Can you work these out from the model? Positions are in its coordinate system, mm. Round coordinates to 2 decimals unless told otherwise and drop trailing zeros. Loops run counter-clockwise (first coordinate to the right, second up) from the corner with the lowest first, then second, coordinate; pieces in that order, holes last.
from build123d import *

# Parameters (mm, degrees)
BOSS_EXTRUDE1_DEPTH = 30
FILLET1_R           = 5
SKETCH2_R           = 14
CUT_EXTRUDE1_DEPTH  = 56.541044473


with BuildPart() as part:
    # Sketch1 → Boss-Extrude1 (new body)
    with BuildSketch(Plane.XY):
        Polygon((0, 40), (34.641016151, -20), (-34.641016151, -20), align=None)
    extrude(amount=BOSS_EXTRUDE1_DEPTH)

    # Fillet1
    fillet1_edges = [part.edges().sort_by_distance(p)[0] for p in [
        (0, 40, 15),
        (34.641016151, -20, 15),
        (-34.641016151, -20, 15),
    ]]
    fillet(fillet1_edges, radius=FILLET1_R)

    # Sketch2 → Cut-Extrude1 (cut, through all)
    with BuildSketch(Plane.XY.offset(30)):
        Circle(SKETCH2_R)
    extrude(amount=-CUT_EXTRUDE1_DEPTH, mode=Mode.SUBTRACT)


solid = part.part
(1) If we section it at D-D, the plane x = 19: List the corners of the cut face in (y, z) for me, then the cut area to 3 significant figures.
Worked answers:
outline: (-20, 0) - (7.09, 0) - (7.09, 30) - (-20, 30) - close
area: 813 mm2
(2) If I drill on line 1 (Y direction, x = 0, z = 9.25); line 2 (Y direction, x = -1, z = 23.5); line 3 (X direction, y = -13, z = 6.5), over which ranges is the centre line in solid material (lowest first)?
Worked answers:
line 1: y = -20 to -14, 14 to 35
line 2: y = -20 to -13.96, 13.96 to 34.9
line 3: x = -30.56 to -5.2, 5.2 to 30.56
(3) If we section it at A-A, the plane x = 0: List the corners of the cut face in (y, z) for me.
Worked answers:
outline: (-20, 0) - (-14, 0) - (-14, 30) - (-20, 30) - close; (14, 0) - (35, 0) - (35, 30) - (14, 30) - close
(4) If we section it at B-B, the plane z = 2: List the corners of the cut face in (x, y) for me, then the cut area to 3 significant figures.
Worked answers:
outline: (-30.31, -12.5) arc R5 ccw to (-25.98, -20) - (25.98, -20) arc R5 ccw to (30.31, -12.5) - (4.33, 32.5) arc R5 ccw to (-4.33, 32.5) - close; hole circle Ø28 at (0, 0)
area: 1,410 mm2
(5) Will these pins go through, and if not, where does the flat tip stop? P1, Ø5, axis at x = 18.5, z = 5.5, coming from the +Y side; P2, Ø1, axis at y = -4, z = 8, coming from the -X side; P3, Ø12, axis at y = 14, z = 5.5, coming from the +X side.
Worked answers:
P1: stops at y = 12.29
P2: stops at x = -25.69
P3: stops at x = 18.48
(6) If we mould it in two halves opening along X, with no side actions, what happens to faces 1 (the flat face through (17.14, 10.31, 14.79)), 2 (the cylindrical face through (-30.274, -17.563, 15.21)), 3 (the cylindrical face through (12.932, -5.362, 15.21))? For each: released by +X, released by -X, zero draft, split by the parting line, or undercut.
Worked answers:
face 1: released by +X
face 2: released by -X
face 3: undercut
(7) If we section it at C-C, the plane y = 0: List the corners of the cut face in (x, z) for me.
Worked answers:
outline: (-23.09, 0) - (-14, 0) - (-14, 30) - (-23.09, 30) - close; (14, 0) - (23.09, 0) - (23.09, 30) - (14, 30) - close
